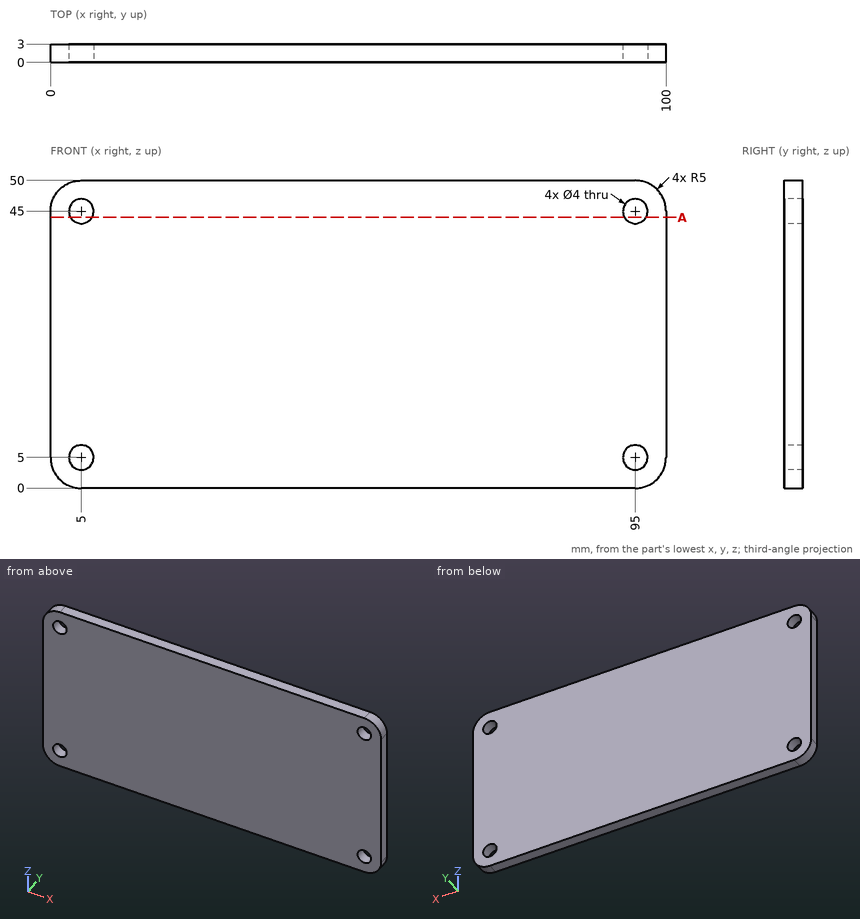
Input: dimensioned drawing with shaded views. Units: mm. Origin: part minimum x, y, z. Give positions to 0.01 mm unless a question says otherwise; leave off trailing zeros. Write each loop counter-clockwise with the first axis right and the second up, starting at its lowest first coordinate (ties: lowest second). Pieces come first, ordered by that corner, then holes.
Q1. Material intervals for probe 1 along Z at (x, y) = (5, 1.6); probe 2 along X at (y, z) = (2.45, 45); probe 3 along Z at (x, y) = (4, 2.3), sorted ascending.
Q2. First-contact query: P1, Ø1, axis at x = 45, z = 17.5, coming from the -Y side; P2, Ø3.5, axis at x = 5, z = 5, coming from the +Y side. Flat tips, straight axial feed; report the tip coordinate or a pass-through.
Q3. Section A-A, the plane z = 44. Output: boundary loops of the cut face in (x, y), plus the area to 3 significant figures.
Filled in:
1. probe 1: z = 0 to 3, 7 to 43, 47 to 50
1. probe 2: x = 0 to 3, 7 to 93, 97 to 100
1. probe 3: z = 0.1 to 3.27, 6.73 to 43.27, 46.73 to 49.9
2. P1: stops at y = 0
2. P2: passes through
3. outline: (0, 0) - (3.27, 0) - (3.27, 3) - (0, 3) - close; (6.73, 0) - (93.27, 0) - (93.27, 3) - (6.73, 3) - close; (96.73, 0) - (100, 0) - (100, 3) - (96.73, 3) - close
3. area: 279 mm2
